from build123d import *

# Parameters (mm, degrees)
SKETCH1_W                = 250
SKETCH1_H                = 100
BOSS_EXTRUDE1_DEPTH      = 4
SKETCH2_W                = 24
SKETCH2_H                = 4
BOSS_EXTRUDE2_DEPTH      = 4
SKETCH3_W                = 4
SKETCH3_H                = 40
SKETCH3_H_2              = 20
CUT_EXTRUDE1_DEPTH       = 5
M4_CLEARANCE_HOLE1_D     = 4.3
M4_CLEARANCE_HOLE1_DEPTH = 6
M4_CLEARANCE_HOLE1_TIP   = 1.291850331
CUT_EXTRUDE2_DEPTH       = 10
SKETCH7_W                = 13
SKETCH7_H                = 5
CUT_EXTRUDE3_DEPTH       = 10


with BuildPart() as part:
    # Sketch1 → Boss-Extrude1 (new body)
    with BuildSketch(Plane.XY):
        Rectangle(SKETCH1_W, SKETCH1_H)
    extrude(amount=BOSS_EXTRUDE1_DEPTH)

    # Sketch2 → Boss-Extrude2 (add)
    with BuildSketch(Plane.XZ.offset(50)):
        with Locations((-78, 2)):
            Rectangle(SKETCH2_W, SKETCH2_H)
        with Locations((-42, 2)):
            Rectangle(SKETCH2_W, SKETCH2_H)
        with Locations((42, 2)):
            Rectangle(SKETCH2_W, SKETCH2_H)
        with Locations((78, 2)):
            Rectangle(SKETCH2_W, SKETCH2_H)
    boss_extrude2 = extrude(amount=BOSS_EXTRUDE2_DEPTH)

    # Sketch3 → Cut-Extrude1 (cut, through all)
    with BuildSketch(Plane.XY.offset(4)):
        with Locations((-8.5, 30)):
            Rectangle(SKETCH3_W, SKETCH3_H)
        with Locations((-8.5, -12)):
            Rectangle(SKETCH3_W, SKETCH3_H_2)
        with Locations((8.5, -12)):
            Rectangle(SKETCH3_W, SKETCH3_H_2)
        with Locations((8.5, 30)):
            Rectangle(SKETCH3_W, SKETCH3_H)
    extrude(amount=-CUT_EXTRUDE1_DEPTH, mode=Mode.SUBTRACT)

    # Mirror1: Boss-Extrude2 across plane
    add(boss_extrude2.mirror(Plane.ZX))

    # M4 Clearance Hole1
    with Locations(Plane.XY.offset(4)):
        with Locations((-8.5, 4), (8.5, 4)):
            Hole(M4_CLEARANCE_HOLE1_D / 2, depth=M4_CLEARANCE_HOLE1_DEPTH)
            with Locations((0, 0, -(M4_CLEARANCE_HOLE1_DEPTH + M4_CLEARANCE_HOLE1_TIP / 2))):  # 118° drill point
                Cone(0, M4_CLEARANCE_HOLE1_D / 2, M4_CLEARANCE_HOLE1_TIP, mode=Mode.SUBTRACT)

    # Sketch6 → Cut-Extrude2 (cut)
    with BuildSketch(Plane.XY.offset(4)):
        Polygon((-62.1, -50), (-57.9, -50), (-57.9, -40), (-55.5, -40), (-55.5, -39), (-56.25, -39), (-56.25, -36.5), (-57.9, -36.5), (-57.9, -33), (-62.1, -33), (-62.1, -36.5), (-63.75, -36.5), (-63.75, -39), (-64.5, -39), (-64.5, -40), (-62.1, -40), align=None)
        Polygon((57.9, -40), (57.9, -50), (62.1, -50), (62.1, -40), (64.5, -40), (64.5, -39), (63.75, -39), (63.75, -36.5), (62.1, -36.5), (62.1, -33), (57.9, -33), (57.9, -36.5), (56.25, -36.5), (56.25, -39), (55.5, -39), (55.5, -40), align=None)
        Polygon((62.1, 40), (62.1, 50), (57.9, 50), (57.9, 40), (55.5, 40), (55.5, 39), (56.25, 39), (56.25, 36.5), (57.9, 36.5), (57.9, 33), (62.1, 33), (62.1, 36.5), (63.75, 36.5), (63.75, 39), (64.5, 39), (64.5, 40), align=None)
        Polygon((-57.9, 50), (-62.1, 50), (-62.1, 40), (-64.5, 40), (-64.5, 39), (-63.75, 39), (-63.75, 36.5), (-62.1, 36.5), (-62.1, 33), (-57.9, 33), (-57.9, 36.5), (-56.25, 36.5), (-56.25, 39), (-55.5, 39), (-55.5, 40), (-57.9, 40), align=None)
    extrude(amount=-CUT_EXTRUDE2_DEPTH, mode=Mode.SUBTRACT)

    # Sketch7 → Cut-Extrude3 (cut)
    with BuildSketch(Plane.XY.offset(4)):
        with Locations((0, 47.5)):
            Rectangle(SKETCH7_W, SKETCH7_H)
    extrude(amount=-CUT_EXTRUDE3_DEPTH, mode=Mode.SUBTRACT)


solid = part.part
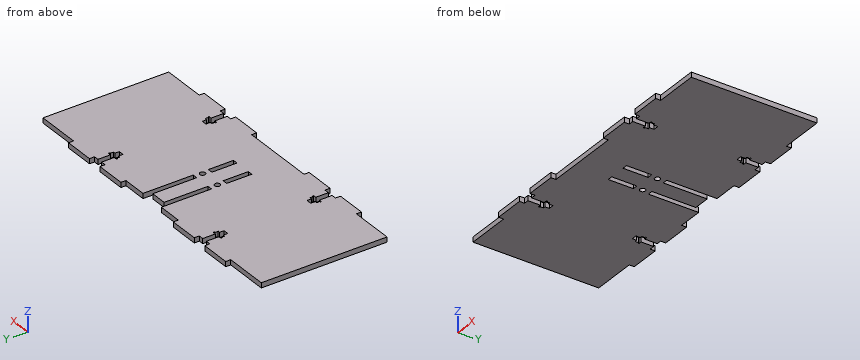
The listing builds one solid part. Answer for the finished solid, in the listing's coordinates (mm). Coordinates: 2 decimals unless noted, no trailing zeros. Loops run counter-clockwise (first coordinate to the right, second up) from the corner with the lowest first, then second, coordinate; pieces in that order, holes last. Notation, with made-up numbers: M 59,88.5 L 106,88.5 A29 cw 106,124.5 Z; hole C 68.25,58 d7. An arc over 180 degrees is marked long. Answer in a Markdown table with one row per item.
1) Find section A-A (y = 30.5). Determine the outline of the cut face in (x, z).
Answers below:
| item | result |
|---|---|
| outline | M -125,0 L -10.5,0 L -10.5,4 L -125,4 Z; M -6.5,0 L 6.5,0 L 6.5,4 L -6.5,4 Z; M 10.5,0 L 125,0 L 125,4 L 10.5,4 Z |
2) Find the intervals of material crossed by probe 1 along X at (y, z) = (17, 3.6); probe 2 along Y at (x, z) = (-8.5, 2.5); probe 3 along X at (y, z) = (43.5, 3.15), in increasing order.
Answers below:
| item | result |
|---|---|
| probe 1 | -125 to -10.5, -6.5 to 6.5, 10.5 to 125 |
| probe 2 | -50 to -22, -2 to 1.85, 6.15 to 10 |
| probe 3 | -125 to -62.1, -57.9 to -10.5, -6.5 to 6.5, 10.5 to 57.9, 62.1 to 125 |
3) Find section B-B (z = 2.35). Count the separate pieces of the cut face and the enclosed holes in it, then the cut area to 3 significant figures.
Answers below:
| item | result |
|---|---|
| separate pieces | 1 |
| enclosed holes | 4 |
| area | 24,900 mm^2 |
4) Given pin 1 (1.2 mm diameter, centred on y = -52.5, z = 2, fed in from -X); pin 2 (1.8 mm diameter, centred on x = -63, z = 2, fed in from +Y); pin 3 (1 mm diameter, centred on x = 61, z = 3.5, fed in from -Y), each flat-ended and moving along its own axis, determine where each tip first touches the part or whether it passes through.
Answers below:
| item | result |
|---|---|
| pin 1 | x = -90 |
| pin 2 | y = 50 |
| pin 3 | y = -33 |
